from build123d import *

# Parameters (mm, degrees)
BOSS_EXTRUDE1_DEPTH = 40
SKETCH2_R           = 2.5
CUT_EXTRUDE1_DEPTH  = 23.5


with BuildPart() as part:
    # Sketch1 → Boss-Extrude1 (new body)
    with BuildSketch(Plane.XY):
        with BuildLine():
            Line((0, 23.5), (0, 0))
            Line((0, 0), (52, 0))
            Line((52, 0), (52, 23.5))
            Line((52, 23.5), (40.924811557, 23.5))
            ThreePointArc((40.924811557, 23.5), (26, 10), (11.075188443, 23.5))
            Line((11.075188443, 23.5), (0, 23.5))
        make_face()
    extrude(amount=BOSS_EXTRUDE1_DEPTH)

    # Sketch2 → Cut-Extrude1 (cut)
    with BuildSketch(Plane(origin=(0, 0, 0), x_dir=(-1, 0, 0), z_dir=(0, -1, 0))):
        with Locations(Location((-6, -8, 0), (0, 0, 90))):
            Circle(SKETCH2_R)
        with Locations(Location((-6, -32, 0), (0, 0, 90))):
            Circle(SKETCH2_R)
        with Locations(Location((-46, -32, 0), (0, 0, 90))):
            Circle(SKETCH2_R)
        with Locations(Location((-46, -8, 0), (0, 0, 90))):
            Circle(SKETCH2_R)
    extrude(amount=-CUT_EXTRUDE1_DEPTH, mode=Mode.SUBTRACT)


solid = part.part
Could you check a few things on this model? Use its own coordinates, in mm. Coordinates: 2 decimals unless noted, no trailing zeros. Loops run counter-clockwise (first coordinate to the right, second up) from the corner with the lowest first, then second, coordinate; pieces in that order, holes last.
1. Imagine slicing it at C-C (y = 18.75). Please give me the cut outline in (x, z).
2. Imagine slicing it at D-D (y = 4.25). Please give me the cut outline in (x, z).
3. Imagine slicing it at A-A (z = 8). Please give me the cut outline in (x, y).
4. Imagine slicing it at B-B (x = 6). Please give me the cut outline in (y, z), and give its area (3 significant figures).
5. We'd pull the mould along Z, two halves only. Please class faces 1 (the face through (26, 0, 20)), 2 (the face through (26, 9, 0)), 3 (the face through (43.56, 11.59, 32.54)): released by +Z, released by -Z, zero draft, split by the parting line, or undercut.
6. I need wall thicknesses on L1, parallel to X at y = 8.25, z = 32; L2, parallel to X at y = 19.5, z = 6; L3, parallel to X at y = 12.5, z = 32. Which ranges of each line are inside material? Lowest first, please.
Computed values:
1. outline: (0, 0) - (12.36, 0) - (12.36, 40) - (0, 40) - close; (39.64, 0) - (52, 0) - (52, 40) - (39.64, 40) - close; hole circle Ø5 at (6, 8); hole circle Ø5 at (6, 32); hole circle Ø5 at (46, 8); hole circle Ø5 at (46, 32)
2. outline: (0, 0) - (52, 0) - (52, 40) - (0, 40) - close; hole circle Ø5 at (6, 8); hole circle Ø5 at (6, 32); hole circle Ø5 at (46, 8); hole circle Ø5 at (46, 32)
3. outline: (0, 0) - (3.5, 0) - (3.5, 23.5) - (0, 23.5) - close; (8.5, 0) - (43.5, 0) - (43.5, 23.5) - (40.92, 23.5) arc R15 cw to (11.08, 23.5) - (8.5, 23.5) - close; (48.5, 0) - (52, 0) - (52, 23.5) - (48.5, 23.5) - close
4. outline: (0, 0) - (23.5, 0) - (23.5, 5.5) - (0, 5.5) - close; (0, 10.5) - (23.5, 10.5) - (23.5, 29.5) - (0, 29.5) - close; (0, 34.5) - (23.5, 34.5) - (23.5, 40) - (0, 40) - close
4. area: 705 mm2
5. face 1: zero draft
5. face 2: released by -Z
5. face 3: undercut
6. L1: x = 0 to 3.5, 8.5 to 43.5, 48.5 to 52
6. L2: x = 0 to 4.5, 7.5 to 12.04, 39.96 to 44.5, 47.5 to 52
6. L3: x = 0 to 3.5, 8.5 to 17.71, 34.29 to 43.5, 48.5 to 52
